Geometry check sheet. Reference: the model listing, model coordinates, mm. A direction names the side the tool comes from. Round coordinates to 2 decimals unless told otherwise and drop trailing zeros. Write each loop counter-clockwise with the first axis right and the second up, starting at its lowest first coordinate (ties: lowest second). Pieces come first, ordered by that corner, then holes. Notation, with made-up numbers: (7, -18) -> (16, -18) arc R11 cw to (16, -4) -> close; hole circle Ø7 at (1.5, 66). An arc over 180 degrees is marked (long way). Use a Markdown table: item, result.
```python
from build123d import *

# Parameters (mm, degrees)
SKETCH_3_R      = 2
SKETCH_3_R_2    = 1.5
EXTRUDE_1_DEPTH = 2


with BuildPart() as part:
    # 草图3 → 凸台-拉伸1 (new body)
    with BuildSketch(Plane.XY):
        with BuildLine():
            Line((-45, -3.990216685), (-28.8, -3.990216685))
            Line((-28.8, -3.990216685), (-28.8, -8.990216685))
            Line((-28.8, -8.990216685), (-24.8, -8.990216685))
            Line((-24.8, -8.990216685), (-24.8, -3.990216685))
            Line((-24.8, -3.990216685), (-14.9, -3.990216685))
            Line((-14.9, -3.990216685), (-14.9, -1.490216685))
            Line((-14.9, -1.490216685), (-16.4, -1.490216685))
            Line((-16.4, -1.490216685), (-16.4, 1.109783315))
            Line((-16.4, 1.109783315), (-14.9, 1.109783315))
            Line((-14.9, 1.109783315), (-14.9, 4.109783315))
            Line((-14.9, 4.109783315), (-11.9, 4.109783315))
            Line((-11.9, 4.109783315), (-11.9, 1.109783315))
            Line((-11.9, 1.109783315), (-10.4, 1.109783315))
            Line((-10.4, 1.109783315), (-10.4, -1.490216685))
            Line((-10.4, -1.490216685), (-11.9, -1.490216685))
            Line((-11.9, -1.490216685), (-11.9, -3.990216685))
            Line((-11.9, -3.990216685), (-2, -3.990216685))
            Line((-2, -3.990216685), (-2, -8.990216685))
            Line((-2, -8.990216685), (0, -8.990216685))
            Line((0, -8.990216685), (2, -8.990216685))
            Line((2, -8.990216685), (2, -3.990216685))
            Line((2, -3.990216685), (11.9, -3.990216685))
            Line((11.9, -3.990216685), (11.9, -1.490216685))
            Line((11.9, -1.490216685), (10.4, -1.490216685))
            Line((10.4, -1.490216685), (10.4, 1.109783315))
            Line((10.4, 1.109783315), (11.9, 1.109783315))
            Line((11.9, 1.109783315), (11.9, 4.109783315))
            Line((11.9, 4.109783315), (14.9, 4.109783315))
            Line((14.9, 4.109783315), (14.9, 1.109783315))
            Line((14.9, 1.109783315), (16.4, 1.109783315))
            Line((16.4, 1.109783315), (16.4, -1.490216685))
            Line((16.4, -1.490216685), (14.9, -1.490216685))
            Line((14.9, -1.490216685), (14.9, -3.990216685))
            Line((14.9, -3.990216685), (24.8, -3.990216685))
            Line((24.8, -3.990216685), (24.8, -8.990216685))
            Line((24.8, -8.990216685), (28.8, -8.990216685))
            Line((28.8, -8.990216685), (28.8, -3.990216685))
            Line((28.8, -3.990216685), (45, -3.990216685))
            Line((45, -3.990216685), (45, 5.009783315))
            Line((45, 5.009783315), (45, 15.009783315))
            Line((45, 15.009783315), (45, 26.463053661))
            Line((45, 26.463053661), (41, 30.009783315))
            Line((41, 30.009783315), (30.874746963, 30.009783315))
            ThreePointArc((30.874746963, 30.009783315), (28.525350528, 27.153364822), (25.912710857, 24.535559602))
            ThreePointArc((25.912710857, 24.535559602), (15.928828372, 14.55206683), (1.809761925, 14.552342399))
            ThreePointArc((1.809761925, 14.552342399), (0, 14.509783315), (-1.809761925, 14.552342399))
            ThreePointArc((-1.809761925, 14.552342399), (-15.928828372, 14.55206683), (-25.912710857, 24.535559602))
            ThreePointArc((-25.912710857, 24.535559602), (-28.525350528, 27.153364822), (-30.874746963, 30.009783315))
            Line((-30.874746963, 30.009783315), (-41, 30.009783315))
            Line((-41, 30.009783315), (-45, 26.463053661))
            Line((-45, 26.463053661), (-45, 15.009783315))
            Line((-45, 15.009783315), (-45, 5.009783315))
            Line((-45, 5.009783315), (-45, -3.990216685))
        make_face()
        with Locations((0, 10.509783315)):
            Circle(SKETCH_3_R, mode=Mode.SUBTRACT)
        with Locations((-30.0520382, 22.957745114)):
            Circle(SKETCH_3_R, mode=Mode.SUBTRACT)
        with Locations((30.0520382, 22.957745114)):
            Circle(SKETCH_3_R, mode=Mode.SUBTRACT)
        with Locations((-26.8, 9.509783315)):
            Circle(SKETCH_3_R_2, mode=Mode.SUBTRACT)
        with Locations(Location((26.8, 9.509783315, 0), (0, 0, 180))):
            Circle(SKETCH_3_R_2, mode=Mode.SUBTRACT)
        with Locations((-42, 10.009783315)):
            Circle(SKETCH_3_R_2, mode=Mode.SUBTRACT)
        with Locations(Location((42, 10.009783315, 0), (0, 0, 180))):
            Circle(SKETCH_3_R_2, mode=Mode.SUBTRACT)
        with BuildLine():
            Line((-43.1, 5.109783315), (-43.1, -0.090216685))
            Line((-43.1, -0.090216685), (-40.9, -0.090216685))
            Line((-40.9, -0.090216685), (-40.9, 5.109783315))
            ThreePointArc((-40.9, 5.109783315), (-42, 5.565418233), (-43.1, 5.109783315))
        make_face(mode=Mode.SUBTRACT)
        with BuildLine():
            Line((-43.1, 20.109783315), (-40.9, 20.109783315))
            Line((-40.9, 20.109783315), (-40.9, 14.909783315))
            ThreePointArc((-40.9, 14.909783315), (-42, 14.454148396), (-43.1, 14.909783315))
            Line((-43.1, 14.909783315), (-43.1, 20.109783315))
        make_face(mode=Mode.SUBTRACT)
        with BuildLine():
            Line((40.9, 20.109783315), (40.9, 14.909783315))
            ThreePointArc((40.9, 14.909783315), (42, 14.454148396), (43.1, 14.909783315))
            Line((43.1, 14.909783315), (43.1, 20.109783315))
            Line((43.1, 20.109783315), (40.9, 20.109783315))
        make_face(mode=Mode.SUBTRACT)
        with BuildLine():
            Line((40.9, 5.109783315), (40.9, -0.090216685))
            Line((40.9, -0.090216685), (43.1, -0.090216685))
            Line((43.1, -0.090216685), (43.1, 5.109783315))
            ThreePointArc((43.1, 5.109783315), (42, 5.565418233), (40.9, 5.109783315))
        make_face(mode=Mode.SUBTRACT)
    extrude(amount=EXTRUDE_1_DEPTH)


solid = part.part
```
(1) Thickness scan on line 1 (X direction, y = 0, z = 0.6); line 2 (X direction, y = -6.5, z = 0.2); line 3 (Y direction, x = 42, z = 0.5). Record the ranges inside material, lowest first.
A:
| item | result |
|---|---|
| line 1 | x = -45 to -43.1, -40.9 to -16.4, -10.4 to 10.4, 16.4 to 40.9, 43.1 to 45 |
| line 2 | x = -28.8 to -24.8, -2 to 2, 24.8 to 28.8 |
| line 3 | y = -3.99 to -0.09, 5.57 to 8.51, 11.51 to 14.45, 20.11 to 29.12 |
(2) Section check B-B on x = 27. Record the cut outline in (y, z), plus the area to 3 significant figures.
A:
| item | result |
|---|---|
| outline | (-8.99, 0) -> (8.02, 0) -> (8.02, 2) -> (-8.99, 2) -> close; (11, 0) -> (25.56, 0) -> (25.56, 2) -> (11, 2) -> close |
| area | 63.2 mm2 |
(3) Access from +Z, -Z, +X, -X, +Y, -Y to the whole of each face (thin tool, end or side, straight path). Record for faces 5 (the face through (-37, -3.99, 1)), 6 (the face through (-16, -1.49, 1)), 7 (the face through (24.8, -6, 1)), 8 (the face through (16.116, 14.631, 0.986)).
A:
| item | result |
|---|---|
| face 5 | +Z, -Z, -X, -Y |
| face 6 | +Z, -Z |
| face 7 | +Z, -Z, -Y |
| face 8 | +Z, -Z, +Y |
(4) Gauge pin test, flat ends, axial feed: pin 1 Ø0.6 at (x, z) = (-13.5, 1.5) entering from -Y; pin 2 Ø0.8 at (x, z) = (-11.5, 1) entering from +Y. Record the tip position at first contact, or that the pin passes through.
A:
| item | result |
|---|---|
| pin 1 | stops at y = 4.11 |
| pin 2 | stops at y = 13.4 |
(5) Section check C-C on y = 16.5. Record the cut outline in (x, z), plus the area to 3 significant figures.
A:
| item | result |
|---|---|
| outline | (-45, 0) -> (-43.1, 0) -> (-43.1, 2) -> (-45, 2) -> close; (-40.9, 0) -> (-19.47, 0) -> (-19.47, 2) -> (-40.9, 2) -> close; (19.47, 0) -> (40.9, 0) -> (40.9, 2) -> (19.47, 2) -> close; (43.1, 0) -> (45, 0) -> (45, 2) -> (43.1, 2) -> close |
| area | 93.3 mm2 |
(6) Section check D-D on x = 42. Record the cut outline in (y, z).
A:
| item | result |
|---|---|
| outline | (-3.99, 0) -> (-0.09, 0) -> (-0.09, 2) -> (-3.99, 2) -> close; (5.57, 0) -> (8.51, 0) -> (8.51, 2) -> (5.57, 2) -> close; (11.51, 0) -> (14.45, 0) -> (14.45, 2) -> (11.51, 2) -> close; (20.11, 0) -> (29.12, 0) -> (29.12, 2) -> (20.11, 2) -> close |
(7) Section check A-A on y = -6. Record the cut outline in (x, z), plus the area to 3 significant figures.
A:
| item | result |
|---|---|
| outline | (-28.8, 0) -> (-24.8, 0) -> (-24.8, 2) -> (-28.8, 2) -> close; (-2, 0) -> (2, 0) -> (2, 2) -> (-2, 2) -> close; (24.8, 0) -> (28.8, 0) -> (28.8, 2) -> (24.8, 2) -> close |
| area | 24.0 mm2 |
(8) Release check for a two-part mould opening along X. For faces 1 (the face through (-28.8, -6, 1)), 2 (the face through (43.5, 9.94, 0.99)), 3 (the face through (-11.9, -3, 1)), 4 (the face through (43.03, 28.21, 0.99)) record: +X half, -X half, draft (parallel to the pull), parting line (faces both ways), or undercut.
A:
| item | result |
|---|---|
| face 1 | -X half |
| face 2 | undercut |
| face 3 | undercut |
| face 4 | +X half |
